from build123d import *

# Parameters (mm, degrees)
F1_DEPTH = 100


with BuildPart() as f1:
    # F0 (on Front) → F1 (new body)
    with BuildSketch(Plane.XZ):
        Polygon((-24.100423, 20), (-24.100423, 0), (-14.100423, 0), (-14.100423, 5), (15.899577, 5), (15.899577, 0), (25.899577, 0), (25.899577, 20), (30.899577, 20), (30.899577, 37), (24.899577, 43), (21.517872, 43), (3.399577, 24.020469), (3.399577, 20), (-1.600423, 20), (-1.600423, 24.020469), (-21.482128, 43), (-23.100423, 43), (-29.100423, 37), (-29.100423, 20), align=None)
    extrude(amount=-F1_DEPTH)


solid = f1.part
Can you work these out from the model? Positions are in its coordinate system, mm. A direction names the side the tool comes from. Give positions to 0.01 mm unless a question says otherwise; leave off trailing zeros. Loops run counter-clockwise (first coordinate to the right, second up) from the corner with the lowest first, then second, coordinate; pieces in that order, holes last. Notation, with made-up numbers: (31.25, -1) - (87.25, -1) arc R32 cw to (87.25, 35) - close; hole circle Ø10 at (16.25, 10.25). An arc over 180 degrees is marked (long way). Return JSON: item names as keys, results as strings.
1. I want a section at D-D on x = 10.5. Please give me the cut outline in (y, z), and give its area (3 significant figures).
Output values:
{"outline": "(0, 5) - (100, 5) - (100, 31.46) - (0, 31.46) - close", "area": "2,650 mm²"}
2. We'd pull the mould along X, two halves only. Please class faces 4 (the face through (-19, 49, 0)), 5 (the face through (15.9, 49, 3)), 6 (the face through (-26.1, 49.3, 40)): +X half, -X half, draft (parallel to the pull), parting line (faces both ways), or undercut.
Output values:
{"face 4": "draft", "face 5": "undercut", "face 6": "-X half"}
3. I want a section at A-A on y = 87.5. Please give me the cut outline in (x, z), and give its area (3 significant figures).
Output values:
{"outline": "(-29.1, 20) - (-24.1, 20) - (-24.1, 0) - (-14.1, 0) - (-14.1, 5) - (15.9, 5) - (15.9, 0) - (25.9, 0) - (25.9, 20) - (30.9, 20) - (30.9, 37) - (24.9, 43) - (21.52, 43) - (3.4, 24.02) - (3.4, 20) - (-1.6, 20) - (-1.6, 24.02) - (-21.48, 43) - (-23.1, 43) - (-29.1, 37) - close", "area": "1,720 mm²"}
4. I'm going to push flat-ended pins straight in: pin 1 Ø5 at (y, z) = (40.5, 10) entering from -X; pin 2 Ø2 at (x, y) = (8.5, 29.5) entering from +Z; pin 3 Ø4 at (y, z) = (74, 16.5) entering from +X. Where does each tip first touch, or does it pass through?
Output values:
{"pin 1": "stops at x = -24.1", "pin 2": "stops at z = 30.41", "pin 3": "stops at x = 25.9"}
5. For faces 1 (the face through (-24.1, 49, 10)), 2 (the face through (28, 49, 20)), 3 (the face through (3.4, 49, 22)), which set-ups out of +Z, -Z, +X, -X, +Y, -Y let a thin tool reach every point of the face, with its end or its side?
Output values:
{"face 1": "-Z, -X, +Y, -Y", "face 2": "-Z, +X, +Y, -Y", "face 3": "+Z, +Y, -Y"}
6. I want a section at B-B on z = 31.5. Please give me the cut outline in (x, y).
Output values:
{"outline": "(-29.1, 0) - (-9.44, 0) - (-9.44, 100) - (-29.1, 100) - close; (10.54, 0) - (30.9, 0) - (30.9, 100) - (10.54, 100) - close"}
7. If I drill on line 1 (X direction, y = 48, z = 16); line 2 (X direction, y = 94.5, z = 38); line 3 (X direction, y = 27, z = 39.5), over which ranges is the centre line in solid material (lowest first)?
Output values:
{"line 1": "x = -24.1 to 25.9", "line 2": "x = -28.1 to -16.24, 16.74 to 29.9", "line 3": "x = -26.6 to -17.82, 18.18 to 28.4"}
8. I want a section at C-C on z = 10.5. Please give me the cut outline in (x, y).
Output values:
{"outline": "(-24.1, 0) - (25.9, 0) - (25.9, 100) - (-24.1, 100) - close"}
